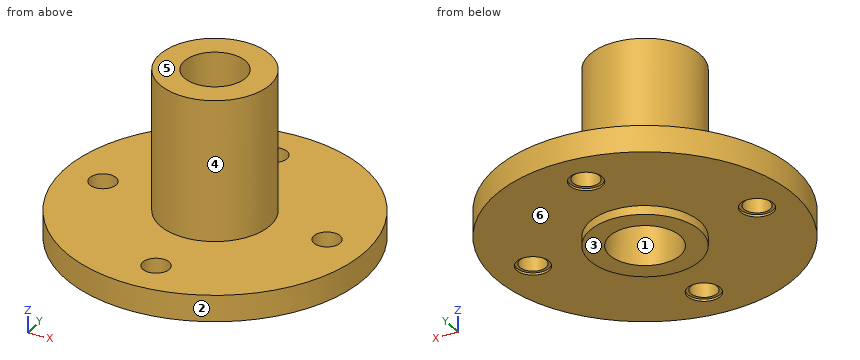
from build123d import *

# Parameters (mm, degrees)
SKETCH1_R           = 17
BOSS_EXTRUDE1_DEPTH = 3
SKETCH2_R           = 1.5
CUT_EXTRUDE1_DEPTH  = 25.228082879
SKETCH3_R           = 6.25
BOSS_EXTRUDE2_DEPTH = 1
BOSS_EXTRUDE3_START = -20
SKETCH5_R           = 6.25
BOSS_EXTRUDE3_DEPTH = 20
SKETCH6_R           = 4
CUT_EXTRUDE2_DEPTH  = 32.272991542
CUT_EXTRUDE2_DRAFT  = -1.5
SKETCH7_R           = 1.85
SKETCH7_R_2         = 1.5
CUT_EXTRUDE3_DEPTH  = 0.25


with BuildPart() as part:
    # Sketch1 → Boss-Extrude1 (new body)
    with BuildSketch(Plane.XY):
        Circle(SKETCH1_R)
    extrude(amount=BOSS_EXTRUDE1_DEPTH)

    # Sketch2 → Cut-Extrude1 (cut, through all)
    with BuildSketch(Plane(origin=(0, 0, 0), x_dir=(-1, 0, 0), z_dir=(0, 0, -1))):
        with Locations((0, 12.5)):
            Circle(SKETCH2_R)
        with Locations((12.5, 0)):
            Circle(SKETCH2_R)
        with Locations((0, -12.5)):
            Circle(SKETCH2_R)
        with Locations((-12.5, 0)):
            Circle(SKETCH2_R)
    extrude(amount=-CUT_EXTRUDE1_DEPTH, mode=Mode.SUBTRACT)

    # Sketch3 → Boss-Extrude2 (add)
    with BuildSketch(Plane(origin=(0, 0, 0), x_dir=(-1, 0, 0), z_dir=(0, 0, -1))):
        with Locations(Location((0, 0, 0), (0, 0, 180))):
            Circle(SKETCH3_R)
    extrude(amount=BOSS_EXTRUDE2_DEPTH)

    # Sketch5 → Boss-Extrude3 (add)
    with BuildSketch(Plane(origin=(0, 0, -1), x_dir=(-1, 0, 0), z_dir=(0, 0, -1)).offset(BOSS_EXTRUDE3_START)):
        with Locations(Location((0, 0, 0), (0, 0, 180))):
            Circle(SKETCH5_R)
    extrude(amount=BOSS_EXTRUDE3_DEPTH)


with BuildPart() as cut_extrude2_tool:
    # Sketch6 → Cut-Extrude2 (with draft: the straight prism first)
    with BuildSketch(Plane(origin=(0, 0, -1), x_dir=(-1, 0, 0), z_dir=(0, 0, -1))):
        Circle(SKETCH6_R)
    extrude(amount=-CUT_EXTRUDE2_DEPTH)
    # Cut-Extrude2: the draft: its side faces are tilted about the plane it starts from
    cut_extrude2_sides = [cut_extrude2_tool.faces().sort_by_distance(p)[0] for p in [
        (4, 0, 15.136495771),
    ]]
    draft(cut_extrude2_sides, Plane(origin=(0, 0, -1), x_dir=(-1, 0, 0), z_dir=(0, 0, -1)), CUT_EXTRUDE2_DRAFT)


with BuildPart() as part_1:
    add(part.part)

    # Cut-Extrude2: cut by cut_extrude2_tool
    add(cut_extrude2_tool.part, mode=Mode.SUBTRACT)

    # Sketch7 → Cut-Extrude3 (cut)
    # profile 1 of 4: a face of its own
    with BuildSketch(Plane(origin=(0, 0, 0), x_dir=(-1, 0, 0), z_dir=(0, 0, -1))):
        with Locations((0, 12.5)):
            Circle(SKETCH7_R)
        with Locations((0, 12.5)):
            Circle(SKETCH7_R_2, mode=Mode.SUBTRACT)
    # profile 2 of 4: a face of its own
    with BuildSketch(Plane(origin=(0, 0, 0), x_dir=(-1, 0, 0), z_dir=(0, 0, -1))):
        with Locations((12.5, 0)):
            Circle(SKETCH7_R)
        with Locations((12.5, 0)):
            Circle(SKETCH7_R_2, mode=Mode.SUBTRACT)
    # profile 3 of 4: a face of its own
    with BuildSketch(Plane(origin=(0, 0, 0), x_dir=(-1, 0, 0), z_dir=(0, 0, -1))):
        with Locations((0, -12.5)):
            Circle(SKETCH7_R)
        with Locations((0, -12.5)):
            Circle(SKETCH7_R_2, mode=Mode.SUBTRACT)
    # profile 4 of 4: a face of its own
    with BuildSketch(Plane(origin=(0, 0, 0), x_dir=(-1, 0, 0), z_dir=(0, 0, -1))):
        with Locations((-12.5, 0)):
            Circle(SKETCH7_R)
        with Locations((-12.5, 0)):
            Circle(SKETCH7_R_2, mode=Mode.SUBTRACT)
    extrude(amount=-CUT_EXTRUDE3_DEPTH, mode=Mode.SUBTRACT)


solid = part_1.part
The listing builds one solid part. Answer for the finished solid, in the listing's coordinates (mm). Face numbers are marked on the shaded views. A direction names the side the tool comes from. Give positions to 0.01 mm unless a question says otherwise; leave off trailing zeros. Order: outer loops, then holes, each group sorted by start corner. A loop starts at its lowest first (then second) coordinate and runs counter-clockwise, first axis right, second up. Notation, with made-up numbers: (7.5, 42) - (15.5, 42) arc R26 cw to (15.5, 77) - close; hole circle Ø5 at (72.25, 88). An arc over 180 degrees is marked (long way). Answer as CSV lines item,"result".
Q1. Straight lines are drawn through the part: L1, parallel to Y at x = 0, z = 1.6; L2, parallel to Z at x = 7, y = -10; L3, parallel to Y at x = 0, z = 0.15. For each, find the intervals that lie inside material, in ascending order.
Answer key:
L1,"y = -17 to -14, -11 to -3.93, 3.93 to 11, 14 to 17"
L2,"z = 0 to 3"
L3,"y = -17 to -14.35, -10.65 to -3.97, 3.97 to 10.65, 14.35 to 17"
Q2. Which of the six approach directions +Z, -Z, +X, -X, +Y, -Y give full straight-line access (tool end or side, diameter ignored) to the marked faces 4, 5 and 6?
Answer key:
face 4,"+Z"
face 5,"+Z, +X, -X, +Y, -Y"
face 6,"-Z"
Q3. Each of these flat-tipped pins is pushed along its axis until it touches: pin 1 Ø3 at (x, y) = (-13.5, 0) entering from -Z; pin 2 Ø6 at (x, y) = (0, -12.5) entering from +Z; pin 3 Ø3.5 at (x, y) = (-12.5, 0) entering from -Z; pin 4 Ø6 at (x, y) = (3.5, 7.5) entering from -Z. Where does it stop, or does it pass through?
Answer key:
pin 1,"stops at z = 0"
pin 2,"stops at z = 3"
pin 3,"stops at z = 0.25"
pin 4,"stops at z = -1"
Q4. A cutting plane is placed at D-D, the plane x = -12.5. Determine the outline of the cut face in (y, z).
Answer key:
outline,"(-11.52, 0) - (-1.85, 0) - (-1.85, 0.25) - (-1.5, 0.25) - (-1.5, 3) - (-11.52, 3) - close; (1.5, 0.25) - (1.85, 0.25) - (1.85, 0) - (11.52, 0) - (11.52, 3) - (1.5, 3) - close"
Q5. A cutting plane is placed at C-C, the plane y = 13.5. Determine the outline of the cut face in (x, z).
Answer key:
outline,"(-10.33, 0) - (-1.56, 0) - (-1.56, 0.25) - (-1.12, 0.25) - (-1.12, 3) - (-10.33, 3) - close; (1.12, 0.25) - (1.56, 0.25) - (1.56, 0) - (10.33, 0) - (10.33, 3) - (1.12, 3) - close"
Q6. A cutting plane is placed at A-A, the plane x = 0. Count the separate pieces of the cut face and the enclosed holes in it, and give its area (3 significant figures).
Answer key:
separate pieces,"4"
enclosed holes,"0"
area,"147 mm^2"
Q7. Determine the mould class of the marked faces 1, 2 and 3 for opening direction X: pulls with the +X half, pulls with the -X half, needs draft (parallel to the pull), parting line crosses it, or undercut.
Answer key:
face 1,"undercut"
face 2,"parting line crosses it"
face 3,"needs draft"
